Input: part model. Units: mm. Frame: model coordinates. Face numbers are marked on the shaded views. A direction names the side the tool comes from. Round coordinates to 2 decimals unless told otherwise and drop trailing zeros. Write each loop counter-clockwise with the first axis right and the second up, starting at its lowest first coordinate (ties: lowest second). Pieces come first, ordered by that corner, then holes. Notation, with made-up numbers: (71.5, 81) - (84.5, 81) arc R12 cw to (84.5, 95) - close; hole circle Ø6 at (49.25, 48). An arc over 180 degrees is marked (long way). Use one line per item in the form item = value.
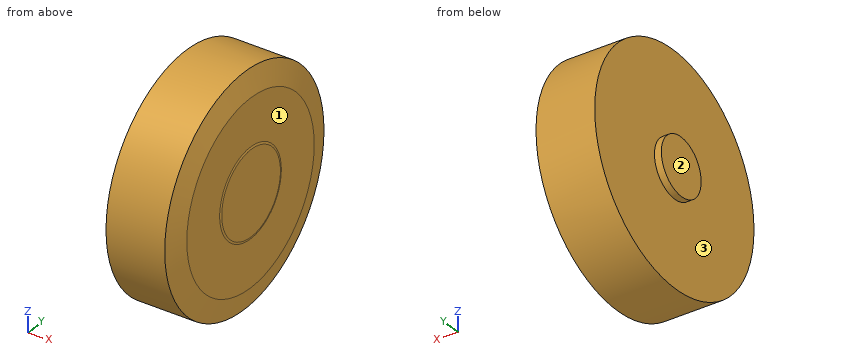
```python
from build123d import *

# Parameters (mm, degrees)
F0_R     = 25.4
F1_DEPTH = 9.652
F2_R     = 4.7625
F3_DEPTH = 4.826
F4_DEPTH = 4.699
F6_DEPTH = 3.175
F7_R     = 6.35
F8_DEPTH = 1.524


# Not quite as in the source:
# - a fillet or chamfer that OpenCascade refuses, or shapes differently, is made with other operations: its cross-section is extruded or revolved along the edge and cut away or added


with BuildPart() as f1:
    # F0 (on Right) → F1 (new body)
    with BuildSketch(Plane.YZ):
        Circle(F0_R)
    extrude(amount=F1_DEPTH)

    # F2 (on face) → F3 (join)
    with BuildSketch(Plane.YZ.offset(9.652)):
        Circle(F2_R)
    extrude(amount=F3_DEPTH)

    # F4 (add): a face of the model
    f4_faces = [f1.faces().sort_by_distance(p)[0] for p in [
        (9.652, -24.6815795103, 0),
    ]]
    extrude(f4_faces, amount=F4_DEPTH)

    # F5: chamfer of 5.08 x 1.3611818976 on 2 edges, made by hand


with BuildPart() as f5_tool2:
    # F5_s3 → F5_t4 (revolve)
    with BuildSketch(Plane.XY):
        Polygon((14.351, 9.8425), (15.7121818976, 4.7625), (14.351, 4.7625), align=None)
    revolve(axis=Axis((14.351, 0, 0), (1, 0, 0)))

    split(bisect_by=Plane.YZ.offset(14.478), keep=Keep.BOTTOM)


with BuildPart() as f1_1:
    add(f1.part)

    # F5_t1: union F5_tool2
    add(f5_tool2.part)

    # F5_s6 → F5_t7 (revolve, cut)
    with BuildSketch(Plane.XY):
        Polygon((12.9898181024, 25.4), (14.351, 20.32), (14.351, 25.4), align=None)
    revolve(axis=Axis((14.351, 0, 0), (1, 0, 0)), mode=Mode.SUBTRACT)

    # F6 (cut): a face of the model
    f6_faces = [f1_1.faces().sort_by_distance(p)[0] for p in [
        (0, 0, 0),
    ]]
    extrude(f6_faces, amount=F6_DEPTH, mode=Mode.SUBTRACT)

    # F7 (on face) → F8 (join)
    with BuildSketch(Plane(origin=(0, 0, 0), x_dir=(0, -1, 0), z_dir=(-1, 0, 0))):
        Circle(F7_R)
    extrude(amount=F8_DEPTH)


solid = f1_1.part
```
(1) Cut plane A-A on z = 0. Output: boundary loops of the cut face in (x, y), then the cut area to 3 significant figures.
Derived:
outline = (-1.52, -6.35) - (0, -6.35) - (0, -25.4) - (12.99, -25.4) - (14.35, -20.32) - (14.35, -9.84) - (14.48, -9.37) - (14.48, 9.37) - (14.35, 9.84) - (14.35, 20.32) - (12.99, 25.4) - (0, 25.4) - (0, 6.35) - (-1.52, 6.35) - close
area = 744 mm^2
(2) Cut plane C-C on x = 5.5. Output: boundary loops of the cut face in (y, z).
Derived:
outline = circle Ø50.8 at (0, 0)
(3) Access query for the marked faces 1, 2 and 3. Directions: +Z, -Z, +X, -X, +Y, -Y. A direction counts if a zero-diameter tool reaches every point of the face in a straight line with its end or side. Return the directions, or none.
Derived:
face_1 = +X
face_2 = +Z, -Z, -X, +Y, -Y
face_3 = -X
(4) Material intervals for L1, parallel to X at y = 7, z = 10.5; L2, parallel to Y at x = 2.25, z = 0.5; L3, parallel to Y at x = 4.75, z = 19, sorted ascending.
Derived:
L1 = 0 to 14.35
L2 = -25.4 to 25.4
L3 = -16.86 to 16.86
(5) First-contact query: pin 1 Ø4 at (x, y) = (12.5, 20.5) entering from +Z; pin 2 Ø1 at (x, z) = (7.5, -9.5) entering from +Y; pin 3 Ø1 at (x, z) = (11.5, 18) entering from -Y; pin 4 Ø4 at (y, z) = (-3.5, 6.5) entering from -X. Flat tips, straight axial feed; report the tip coordinate or a pass-through.
Derived:
pin_1 = 17.4
pin_2 = 23.75
pin_3 = -18.41
pin_4 = -1.52
